Design review of the part built by this model. Coordinates are the model's own, in mm. A direction names the side the tool comes from. Coordinates: 2 decimals unless noted, no trailing zeros. Write each loop counter-clockwise with the first axis right and the second up, starting at its lowest first coordinate (ties: lowest second). Pieces come first, ordered by that corner, then holes. Notation, with made-up numbers: M 33,47.5 L 77,47.5 A29 ccw 77,79.5 Z; hole C 84,62.5 d5. An arc over 180 degrees is marked long. Return JSON: item names as keys, results as strings. Group by question number.
```python
from build123d import *

# Parameters (mm, degrees)
SKETCH1_W           = 30
SKETCH1_H           = 25
BOSS_EXTRUDE1_DEPTH = 1
SKETCH2_W           = 1
SKETCH2_H           = 25
BOSS_EXTRUDE2_DEPTH = 25
BOSS_EXTRUDE3_DEPTH = 1
SKETCH7_R           = 1.5
CUT_EXTRUDE1_DEPTH  = 3


with BuildPart() as part:
    # Sketch1 → Boss-Extrude1 (new body)
    with BuildSketch(Plane.XY):
        Rectangle(SKETCH1_W, SKETCH1_H)
    extrude(amount=BOSS_EXTRUDE1_DEPTH)

    # Sketch2 → Boss-Extrude2 (add)
    with BuildSketch(Plane.XY.offset(1)):
        with Locations((14.5, 0)):
            Rectangle(SKETCH2_W, SKETCH2_H)
    extrude(amount=BOSS_EXTRUDE2_DEPTH)

    # Sketch6 → Boss-Extrude3 (add)
    with BuildSketch(Plane.XZ.offset(12.5)):
        Polygon((14, 26), (-15, 1), (14, 1), align=None)
    boss_extrude3 = extrude(amount=-BOSS_EXTRUDE3_DEPTH)

    # Mirror2: Boss-Extrude3 across plane
    add(boss_extrude3.mirror(Plane.ZX))

    # Sketch7 → Cut-Extrude1 (cut)
    with BuildSketch(Plane.ZY.offset(-14)):
        with Locations(Location((11, 0, 0), (0, 0, 270))):
            Circle(SKETCH7_R)
    extrude(amount=-CUT_EXTRUDE1_DEPTH, mode=Mode.SUBTRACT)


solid = part.part
```
Item 1: Add section D-D (x = -11.5). Write out the cut boundary in (y, z).
Item 2: Add section A-A (y = 0). Write out the cut boundary in (x, z), plus the area to 3 significant figures.
Item 3: For pin 1 (7 mm diameter, centred on y = 3, z = 8.5, fed in from -X), flat-tipped, find the tip position at first contact; note if it passes through.
Item 4: For line 1 (Y direction, x = 13.5, z = 1.5); line 2 (Z direction, x = 14.65, y = 0); line 3 (Z direction, x = -9.5, y = 10.25), list the stretches that pass through material, from the lowest coordinate up.
Item 5: Add section B-B (z = 1.75). Write out the cut boundary in (x, y), plus the area to 3 significant figures.
Item 6: The part is to be moulded in two halves that separate along Y. For faces 3 (the cylindrical face through (14.49, -1.43, 11.45)), 4 (the flat face through (15, 0, 13)), 5 (the flat face through (3, -12.5, 10)), 6 (the flat face through (-1, 0, 1)), say which applies: pulls with the +Y half, pulls with the -Y half, needs draft (parallel to the pull), parting line crosses it, or undercut.
Item 7: Machinability: for faces 1 (the flat face through (-0.3, -12.01, 13.67)), 2 (the flat face through (6, 11.5, 8)), which of the approach directions +Z, -Z, +X, -X, +Y, -Y give a long, thin tool a straight path to every point of the face, cutting with its end or side? Answer none if there is none.
Item 8: Add section C-C (z = 11.75). Write out the cut boundary in (x, y).
Geometry check:
{
 "1": {"outline": "M -12.5,0 L 12.5,0 L 12.5,4.02 L 11.5,4.02 L 11.5,1 L -11.5,1 L -11.5,4.02 L -12.5,4.02 Z"},
 "2": {"outline": "M -15,0 L 15,0 L 15,9.5 L 14,9.5 L 14,1 L -15,1 Z; M 14,12.5 L 15,12.5 L 15,26 L 14,26 Z", "area": "52.0 mm^2"},
 "3": {"pin 1": "x = 14"},
 "4": {"line 1": "-12.5 to -11.5, 11.5 to 12.5", "line 2": "0 to 9.5, 12.5 to 26", "line 3": "0 to 1"},
 "5": {"outline": "M -14.13,-12.5 L 15,-12.5 L 15,12.5 L -14.13,12.5 L -14.13,11.5 L 14,11.5 L 14,-11.5 L -14.13,-11.5 Z", "area": "81.3 mm^2"},
 "6": {"face 3": "undercut", "face 4": "needs draft", "face 5": "pulls with the -Y half", "face 6": "undercut"},
 "7": {"face 1": "+Z, -X, +Y, -Y", "face 2": "+Z, -X"},
 "8": {"outline": "M -2.53,-12.5 L 15,-12.5 L 15,-1.3 L 14,-1.3 L 14,-11.5 L -2.53,-11.5 Z; M -2.53,11.5 L 14,11.5 L 14,1.3 L 15,1.3 L 15,12.5 L -2.53,12.5 Z"}
}
